```python
from build123d import *

# Parameters (mm, degrees)
ESBO_O1_W                        = 64
ESBO_O1_H                        = 39
FLANGE_BASE1_DEPTH               = 3
ESBO_O6_R                        = 2
ESBO_O6_R_2                      = 2.5
ESBO_O6_R_3                      = 0.75
CORTE_EXTRUS_O1_DEPTH            = 10
ARESTA_FLANGE1_STRIP_W           = 13.4732
ARESTA_FLANGE1_STRIP_H           = 3
ARESTA_FLANGE1_STRIP_CUT_DEPTH   = 39
ARESTA_FLANGE1_STRIP_2_W         = 13.4732
ARESTA_FLANGE1_STRIP_2_H         = 3
ARESTA_FLANGE1_STRIP_CUT_2_DEPTH = 39
ARESTA_FLANGE1_DEPTH             = 39
ARESTA_FLANGE1_BEND_DEPTH        = 39
CORTE_EXTRUS_O2_REACH            = 80.845
ESBO_O13_R                       = 2
FILETE1_R                        = 5
ESBO_O13_3_R                     = 2
CUT_EXTRUDE1_DEPTH               = 2
BOSS_EXTRUDE1_DEPTH              = 0.5
SKETCH15_W                       = 17.2634
SKETCH15_H                       = 27
CUT_EXTRUDE2_DEPTH               = 3
FILLET1_R                        = 5
CUT_EXTRUDE3_START               = -70
CUT_EXTRUDE3_DEPTH               = 70
FILLET2_R                        = 3


# Sheet-metal steps are written as plain solids
with BuildPart() as part:
    # Esboço1 → Flange-base1 (new body)
    with BuildSketch(Plane.XY):
        with Locations((-5.006264217, -4.490936556)):
            Rectangle(ESBO_O1_W, ESBO_O1_H)
    extrude(amount=-FLANGE_BASE1_DEPTH)

    # Esboço6 → Corte-extrusão1 (cut)
    with BuildSketch(Plane.XY):
        with Locations((-21.056264217, 6.009063444)):
            Circle(ESBO_O6_R)
        with Locations((-21.056264217, -14.990936556)):
            Circle(ESBO_O6_R)
        with Locations((-5.006264217, -4.490936556)):
            Circle(ESBO_O6_R_2)
        with Locations((-5.006264217, -12.940936556)):
            Circle(ESBO_O6_R_3)
        with Locations((-5.006264217, 3.959063444)):
            Circle(ESBO_O6_R_3)
    extrude(amount=-CORTE_EXTRUS_O1_DEPTH, mode=Mode.SUBTRACT)

    # Aresta-Flange1 strip (across the edge) → Aresta-Flange1 strip cut (cut)
    with BuildSketch(Plane(origin=(26.993735783, -23.990936556, 0), x_dir=(-1, 0, 0), z_dir=(0, 1, 0))):
        with Locations((-6, -1.5)):
            Rectangle(ARESTA_FLANGE1_STRIP_W, ARESTA_FLANGE1_STRIP_H)
    extrude(amount=ARESTA_FLANGE1_STRIP_CUT_DEPTH, mode=Mode.SUBTRACT)

    # Aresta-Flange1 strip 2 (across the edge) → Aresta-Flange1 strip cut 2 (cut)
    with BuildSketch(Plane(origin=(-37.006264217, 15.009063444, 0), x_dir=(1, 0, 0), z_dir=(0, -1, 0))):
        with Locations((-6, -1.5)):
            Rectangle(ARESTA_FLANGE1_STRIP_2_W, ARESTA_FLANGE1_STRIP_2_H)
    extrude(amount=ARESTA_FLANGE1_STRIP_CUT_2_DEPTH, mode=Mode.SUBTRACT)

    # Aresta-Flange1 section (across the edge) → Aresta-Flange1 (add)
    with BuildSketch(Plane(origin=(26.993735783, -23.990936556, 0), x_dir=(-1, 0, 0), z_dir=(0, 1, 0))):
        with BuildLine():
            Line((-3, 0.7366), (-3, 27.22))
            Line((-3, 27.22), (0, 27.22))
            Line((0, 27.22), (0, 0.7366))
            ThreePointArc((0, 0.7366), (0.215745145, 0.215745145), (0.7366, 0))
            Line((0.7366, 0), (0.7366, -3))
            ThreePointArc((0.7366, -3), (-1.905575199, -1.905575199), (-3, 0.7366))
        make_face()
    extrude(amount=ARESTA_FLANGE1_DEPTH)

    # Aresta-Flange1 section 2 (across the edge) → Aresta-Flange1 bend (add)
    with BuildSketch(Plane(origin=(-37.006264217, 15.009063444, 0), x_dir=(1, 0, 0), z_dir=(0, -1, 0))):
        with BuildLine():
            Line((-3, 0.7366), (-3, 27.22))
            Line((-3, 27.22), (0, 27.22))
            Line((0, 27.22), (0, 0.7366))
            ThreePointArc((0, 0.7366), (0.215745145, 0.215745145), (0.7366, 0))
            Line((0.7366, 0), (0.7366, -3))
            ThreePointArc((0.7366, -3), (-1.905575199, -1.905575199), (-3, 0.7366))
        make_face()
    extrude(amount=ARESTA_FLANGE1_BEND_DEPTH)

    # Corte-extrusão2: up to this face of the body (flat: up to its plane)
    corte_extrus_o2_end = Plane(part.part.faces().sort_by_distance((29.993735783, -4.490936556, 13.9783))[0])
    # Esboço13 → Corte-extrusão2 (cut, up to the picked face)
    with BuildSketch(Plane.ZY.offset(40.006264217), mode=Mode.PRIVATE) as corte_extrus_o2_sk1:
        with Locations((21.86, -8.287001978)):
            Circle(ESBO_O13_R)
    corte_extrus_o2_tool1 = split(extrude(corte_extrus_o2_sk1.sketch, amount=-CORTE_EXTRUS_O2_REACH, mode=Mode.PRIVATE), bisect_by=corte_extrus_o2_end, keep=Keep.BOTH, mode=Mode.PRIVATE)
    # Esboço13 → Corte-extrusão2 (cut, up to the picked face)
    with BuildSketch(Plane.ZY.offset(40.006264217), mode=Mode.PRIVATE) as corte_extrus_o2_sk2:
        Polygon((27.22, -11.990936556), (0.7366, -23.990936556), (27.22, -23.990936556), align=None)
    corte_extrus_o2_tool2 = split(extrude(corte_extrus_o2_sk2.sketch, amount=-CORTE_EXTRUS_O2_REACH, mode=Mode.PRIVATE), bisect_by=corte_extrus_o2_end, keep=Keep.BOTH, mode=Mode.PRIVATE)
    add(corte_extrus_o2_tool1.solids().sort_by(Axis((-40.006264, -8.287002, 21.86), (1, 0, 0)))[0], mode=Mode.SUBTRACT)
    add(corte_extrus_o2_tool2.solids().sort_by(Axis((-40.006264, -19.990937, 18.3922), (1, 0, 0)))[0], mode=Mode.SUBTRACT)

    # Filete1
    filete1_edges = [part.edges().sort_by_distance(p)[0] for p in [
        (-38.506264217, -11.990936556, 27.22),
        (28.493735783, -11.990936556, 27.22),
        (28.493735783, 15.009063444, 27.22),
        (-38.506264217, 15.009063444, 27.22),
    ]]
    fillet(filete1_edges, radius=FILETE1_R)

    # Esboço13<3> → Cut-Extrude1 (cut)
    with BuildSketch(Plane.ZY.offset(40.006264217)):
        Polygon((21.86, -3.668199824), (17.86, -5.977600901), (17.86, -10.596403054), (21.86, -12.905804131), (25.86, -10.596403054), (25.86, -5.977600901), align=None)
        with Locations((21.86, -8.287001978)):
            Circle(ESBO_O13_3_R, mode=Mode.SUBTRACT)
    cut_extrude1 = extrude(amount=-CUT_EXTRUDE1_DEPTH, mode=Mode.SUBTRACT)

    # Sketch7 → Boss-Extrude1 (add)
    with BuildSketch(Plane(origin=(-37.006264217, 0, 0), x_dir=(0, 0, -1), z_dir=(1, 0, 0))):
        with BuildLine():
            ThreePointArc((-23.546022833, -13.522202738), (-23.915908256, -13.425840182), (-24.283610421, -13.32145586))
            Line((-24.283610421, -13.32145586), (-22.170433783, -14.278965835))
            ThreePointArc((-22.170433783, -14.278965835), (-16.672492687, -5.272077786), (-27.22, -5.59063405))
            Line((-27.22, -5.59063405), (-27.22, -7.053956966))
            ThreePointArc((-27.22, -7.053956966), (-17.36732716, -5.11432318), (-22.490825712, -13.750705751))
            ThreePointArc((-22.490825712, -13.750705751), (-23.024044759, -13.66240892), (-23.546022833, -13.522202738))
        make_face()
    boss_extrude1 = extrude(amount=BOSS_EXTRUDE1_DEPTH)

    # Mirror1: Cut-Extrude1, Boss-Extrude1 across plane
    add(cut_extrude1.mirror(Plane.ZY.offset(5.006264217)), mode=Mode.SUBTRACT)
    add(boss_extrude1.mirror(Plane.ZY.offset(5.006264217)))

    # Sketch15 → Cut-Extrude2 (cut)
    with BuildSketch(Plane.XY):
        with Locations((11.625435783, -4.490936556)):
            Rectangle(SKETCH15_W, SKETCH15_H)
    extrude(amount=-CUT_EXTRUDE2_DEPTH, mode=Mode.SUBTRACT)

    # Fillet1
    fillet1_edges = [part.edges().sort_by_distance(p)[0] for p in [
        (2.993735783, -17.990936556, -1.5),
        (2.993735783, 9.009063444, -1.5),
        (20.257135783, 9.009063444, -1.5),
        (20.257135783, -17.990936556, -1.5),
    ]]
    fillet(fillet1_edges, radius=FILLET1_R)

    # Sketch16 → Cut-Extrude3 (cut)
    with BuildSketch(Plane(origin=(29.993735783, 0, 0), x_dir=(0, 0, -1), z_dir=(1, 0, 0)).offset(CUT_EXTRUDE3_START)):
        with BuildLine():
            Line((-21.22, 9.009063444), (-3.7366, 9.009063444))
            Line((-3.7366, 9.009063444), (-3.7366, -16.044391464))
            Line((-3.7366, -16.044391464), (-12.588351652, -12.033538634))
            ThreePointArc((-12.588351652, -12.033538634), (-13.394705743, -2.963582668), (-21.22, 1.692497008))
            Line((-21.22, 1.692497008), (-21.22, 9.009063444))
        make_face()
    extrude(amount=CUT_EXTRUDE3_DEPTH, mode=Mode.SUBTRACT)

    # Fillet2
    fillet2_edges = [part.edges().sort_by_distance(p)[0] for p in [
        (28.493735783, 1.692497008, 21.22),
        (28.493735783, 9.009063444, 21.22),
        (28.493735783, 9.009063444, 3.7366),
        (28.493735783, -16.044391464, 3.7366),
        (28.493735783, -12.033538634, 12.588351652),
        (-38.506264217, 1.692497008, 21.22),
        (-38.506264217, 9.009063444, 21.22),
        (-38.506264217, 9.009063444, 3.7366),
        (-38.506264217, -16.044391464, 3.7366),
        (-38.506264217, -12.033538634, 12.588351652),
    ]]
    fillet(fillet2_edges, radius=FILLET2_R)


solid = part.part
```
Geometry: final body of the model. Coordinates: model frame, mm. A direction names the side the tool comes from. Round coordinates to 2 decimals unless told otherwise and drop trailing zeros. Loops run counter-clockwise (first coordinate to the right, second up) from the corner with the lowest first, then second, coordinate; pieces in that order, holes last.
Item 1: Section A-A, the plane x = 5.5. Output: boundary loops of the cut face in (y, z), plus the area to 3 significant figures.
Checked values:
outline: (-23.99, -3) - (-17.32, -3) - (-17.32, 0) - (-23.99, 0) - close; (8.34, -3) - (15.01, -3) - (15.01, 0) - (8.34, 0) - close
area: 40.0 mm2
Item 2: Section B-B, the plane z = 2. Output: boundary loops of the cut face in (x, y), plus the area to 3 significant figures.
Checked values:
outline: (-40.01, -23.42) - (-37.01, -23.42) - (-37.01, 15.01) - (-40.01, 15.01) - close; (26.99, -23.42) - (29.99, -23.42) - (29.99, 15.01) - (26.99, 15.01) - close
area: 231 mm2
Item 3: Reachability of faces 5 (the flat face through (-39.02, -4.84, 23.89)), 6 (the flat face through (2.994, -5, -1)), 7 (the flat face through (29, -8, 25.86)) from +Z, -Z, +X, -X, +Y, -Y: full face, straight path, thin tool, end or side. Return the list, or none.
Checked values:
face 5: -X
face 6: +Z, -Z
face 7: +X
Item 4: Section C-C, the plane y = 11. Output: boundary loops of the cut face in (x, z), plus the area to 3 significant figures.
Checked values:
outline: (-40.01, 0.74) arc R3.74 ccw to (-36.27, -3) - (26.26, -3) arc R3.74 ccw to (29.99, 0.74) - (29.99, 27.12) - (26.99, 27.12) - (26.99, 0.74) arc R0.74 cw to (26.26, 0) - (-36.27, 0) arc R0.74 cw to (-37.01, 0.74) - (-37.01, 27.12) - (-40.01, 27.12) - close
area: 367 mm2
Item 5: Contact query for flat-ended pins moving along their axis: P1, Ø6.5, axis at y = -8.29, z = 21.86, coming from the -X side; P2, Ø5.5, axis at y = -7, z = 21, coming from the +X side; P3, Ø0.6, axis at x = 29.5, y = -9.5, coming from the +Z side; P4, Ø2.5, axis at y = -7.5, z = 23.5, coming from the +X side. Output: stop coordinate, or through.
Checked values:
P1: stops at x = -38.01
P2: stops at x = 29.99
P3: stops at z = 27.2
P4: stops at x = 27.99
Item 6: Line query: L1, parallel to X at y = -6, z = 17; L2, parallel to Z at x = -25, y = 1; L3, parallel to Y at x = 27.5, z = 21.86. Output: solid intervals per line, ascending.
Checked values:
L1: x = -40.01 to -37.01, 26.99 to 29.99
L2: z = -3 to 0
L3: y = -14.42 to -10.29, -6.29 to 15.01
Item 7: Mould query, pull axis Z, two halves, no side actions, for faces 1 (the flat face through (12, -17.991, -1)), 2 (the flat face through (28, 9.009, 13)), 3 (the flat face through (-37.006, -4, 14)), 4 (the cylindrical face through (28.87, -4.764, -1.934)). Classes: released by +Z, released by -Z, zero draft, split by the parting line, or undercut.
Checked values:
face 1: zero draft
face 2: undercut
face 3: undercut
face 4: released by -Z
